from build123d import *

# Parameters (mm, degrees)
CROQUIS1_W              = 220
CROQUIS1_H              = 320
CROQUIS1_R              = 1.55
CROQUIS1_R_2            = 1.575
SALIENTE_EXTRUIR1_DEPTH = 3
CROQUIS2_OUTSIDE_W      = 299.668
CROQUIS2_OUTSIDE_H      = 399.668
CORTAR_EXTRUIR1_DEPTH   = 3
REDONDEO1_R             = 3


with BuildPart() as part:
    # Croquis1 → Saliente-Extruir1 (new body)
    with BuildSketch(Plane(origin=(0, 0, 0), x_dir=(1, 0, 0), z_dir=(0, 1, 0))):
        with Locations((110, 160)):
            Rectangle(CROQUIS1_W, CROQUIS1_H)
        with Locations((185, 167.5)):
            Circle(CROQUIS1_R, mode=Mode.SUBTRACT)
        with Locations((205, 167.5)):
            Circle(CROQUIS1_R, mode=Mode.SUBTRACT)
        with Locations((185, 152.5)):
            Circle(CROQUIS1_R, mode=Mode.SUBTRACT)
        with Locations((205, 152.5)):
            Circle(CROQUIS1_R, mode=Mode.SUBTRACT)
        with Locations((35, 215.5)):
            Circle(CROQUIS1_R_2, mode=Mode.SUBTRACT)
        with Locations((35, 200.5)):
            Circle(CROQUIS1_R_2, mode=Mode.SUBTRACT)
        with Locations((35, 119.5)):
            Circle(CROQUIS1_R_2, mode=Mode.SUBTRACT)
        with Locations((35, 104.5)):
            Circle(CROQUIS1_R_2, mode=Mode.SUBTRACT)
        with Locations((5.5, 314.5)):
            Circle(CROQUIS1_R_2, mode=Mode.SUBTRACT)
        with Locations((214.5, 314.5)):
            Circle(CROQUIS1_R_2, mode=Mode.SUBTRACT)
        with Locations((214.5, 5.5)):
            Circle(CROQUIS1_R_2, mode=Mode.SUBTRACT)
        with Locations((5.5, 5.5)):
            Circle(CROQUIS1_R_2, mode=Mode.SUBTRACT)
        with Locations((15, 200.5)):
            Circle(CROQUIS1_R_2, mode=Mode.SUBTRACT)
        with Locations((15, 215.5)):
            Circle(CROQUIS1_R_2, mode=Mode.SUBTRACT)
        with Locations((15, 104.5)):
            Circle(CROQUIS1_R_2, mode=Mode.SUBTRACT)
        with Locations((15, 119.5)):
            Circle(CROQUIS1_R_2, mode=Mode.SUBTRACT)
        with Locations((110, 180)):
            Circle(CROQUIS1_R_2, mode=Mode.SUBTRACT)
        with Locations((110, 140)):
            Circle(CROQUIS1_R_2, mode=Mode.SUBTRACT)
        with Locations((185, 104.5)):
            Circle(CROQUIS1_R_2, mode=Mode.SUBTRACT)
        with Locations((205, 104.5)):
            Circle(CROQUIS1_R_2, mode=Mode.SUBTRACT)
        with Locations((205, 119.5)):
            Circle(CROQUIS1_R_2, mode=Mode.SUBTRACT)
        with Locations((185, 119.5)):
            Circle(CROQUIS1_R_2, mode=Mode.SUBTRACT)
        with Locations((185, 200.5)):
            Circle(CROQUIS1_R_2, mode=Mode.SUBTRACT)
        with Locations((185, 215.5)):
            Circle(CROQUIS1_R_2, mode=Mode.SUBTRACT)
        with Locations((205, 200.5)):
            Circle(CROQUIS1_R_2, mode=Mode.SUBTRACT)
        with Locations((205, 215.5)):
            Circle(CROQUIS1_R_2, mode=Mode.SUBTRACT)
        with Locations((5.5, 160)):
            Circle(CROQUIS1_R_2, mode=Mode.SUBTRACT)
        with Locations((35, 152.5)):
            Circle(CROQUIS1_R, mode=Mode.SUBTRACT)
        with Locations((15, 152.5)):
            Circle(CROQUIS1_R, mode=Mode.SUBTRACT)
        with Locations((15, 167.5)):
            Circle(CROQUIS1_R, mode=Mode.SUBTRACT)
        with Locations((35, 167.5)):
            Circle(CROQUIS1_R, mode=Mode.SUBTRACT)
        with Locations((214.5, 160)):
            Circle(CROQUIS1_R_2, mode=Mode.SUBTRACT)
    extrude(amount=SALIENTE_EXTRUIR1_DEPTH)

    # Croquis2 outside → Cortar-Extruir1 (cut)
    with BuildSketch(Plane(origin=(0, 3, 0), x_dir=(1, 0, 0), z_dir=(0, 1, 0))):
        with Locations((110, 160)):
            Rectangle(CROQUIS2_OUTSIDE_W, CROQUIS2_OUTSIDE_H)
        with BuildLine():
            Line((9, 148.77502784), (9, 94.5))
            Line((9, 94.5), (19, 94.5))
            Line((19, 94.5), (19, 30))
            Line((19, 30), (1.298802547, 9.049639413))
            ThreePointArc((1.298802547, 9.049639413), (1.950360587, 1.298802547), (9.701197453, 1.950360587))
            Line((9.701197453, 1.950360587), (24.106631311, 19))
            Line((24.106631311, 19), (195.893368689, 19))
            Line((195.893368689, 19), (210.298802547, 1.950360587))
            ThreePointArc((210.298802547, 1.950360587), (218.049639413, 1.298802547), (218.701197453, 9.049639413))
            Line((218.701197453, 9.049639413), (201, 30))
            Line((201, 30), (201, 94.5))
            Line((201, 94.5), (211, 94.5))
            Line((211, 94.5), (211, 148.77502784))
            ThreePointArc((211, 148.77502784), (212.318863014, 152.528287293), (215.695652174, 154.631535054))
            ThreePointArc((215.695652174, 154.631535054), (220, 160), (215.695652174, 165.368464946))
            ThreePointArc((215.695652174, 165.368464946), (212.318863014, 167.471712707), (211, 171.22497216))
            Line((211, 171.22497216), (211, 225.5))
            Line((211, 225.5), (201, 225.5))
            Line((201, 225.5), (201, 290))
            Line((201, 290), (218.701197453, 310.950360587))
            ThreePointArc((218.701197453, 310.950360587), (218.049639413, 318.701197453), (210.298802547, 318.049639413))
            Line((210.298802547, 318.049639413), (195.893368689, 301))
            Line((195.893368689, 301), (24.106631311, 301))
            Line((24.106631311, 301), (9.701197453, 318.049639413))
            ThreePointArc((9.701197453, 318.049639413), (1.950360587, 318.701197453), (1.298802547, 310.950360587))
            Line((1.298802547, 310.950360587), (19, 290))
            Line((19, 290), (19, 225.5))
            Line((19, 225.5), (9, 225.5))
            Line((9, 225.5), (9, 171.22497216))
            ThreePointArc((9, 171.22497216), (7.681136986, 167.471712707), (4.304347826, 165.368464946))
            ThreePointArc((4.304347826, 165.368464946), (0, 160), (4.304347826, 154.631535054))
            ThreePointArc((4.304347826, 154.631535054), (7.681136986, 152.528287293), (9, 148.77502784))
        make_face(mode=Mode.SUBTRACT)
        with BuildLine():
            Line((182, 276), (182, 246))
            ThreePointArc((182, 246), (179.071067812, 238.928932188), (172, 236))
            Line((172, 236), (118, 236))
            ThreePointArc((118, 236), (116.585786438, 236.585786438), (116, 238))
            Line((116, 238), (116, 284))
            ThreePointArc((116, 284), (116.585786438, 285.414213562), (118, 286))
            Line((118, 286), (172, 286))
            ThreePointArc((172, 286), (179.071067812, 283.071067812), (182, 276))
        make_face()
        with BuildLine():
            Line((102, 286), (48, 286))
            ThreePointArc((48, 286), (40.928932188, 283.071067812), (38, 276))
            Line((38, 276), (38, 246))
            ThreePointArc((38, 246), (40.928932188, 238.928932188), (48, 236))
            Line((48, 236), (102, 236))
            ThreePointArc((102, 236), (103.414213562, 236.585786438), (104, 238))
            Line((104, 238), (104, 284))
            ThreePointArc((104, 284), (103.414213562, 285.414213562), (102, 286))
        make_face()
        with BuildLine():
            Line((102, 84), (48, 84))
            ThreePointArc((48, 84), (40.928932188, 81.071067812), (38, 74))
            Line((38, 74), (38, 44))
            ThreePointArc((38, 44), (40.928932188, 36.928932188), (48, 34))
            Line((48, 34), (102, 34))
            ThreePointArc((102, 34), (103.414213562, 34.585786438), (104, 36))
            Line((104, 36), (104, 82))
            ThreePointArc((104, 82), (103.414213562, 83.414213562), (102, 84))
        make_face()
        with BuildLine():
            Line((116, 36), (116, 82))
            ThreePointArc((116, 82), (116.585786438, 83.414213562), (118, 84))
            Line((118, 84), (172, 84))
            ThreePointArc((172, 84), (179.071067812, 81.071067812), (182, 74))
            Line((182, 74), (182, 44))
            ThreePointArc((182, 44), (179.071067812, 36.928932188), (172, 34))
            Line((172, 34), (118, 34))
            ThreePointArc((118, 34), (116.585786438, 34.585786438), (116, 36))
        make_face()
        with BuildLine():
            Line((55, 152), (55, 119))
            ThreePointArc((55, 119), (57.928932188, 111.928932188), (65, 109))
            Line((65, 109), (85, 109))
            ThreePointArc((85, 109), (92.071067812, 111.928932188), (95, 119))
            Line((95, 119), (95, 152))
            ThreePointArc((95, 152), (94.414213562, 153.414213562), (93, 154))
            Line((93, 154), (57, 154))
            ThreePointArc((57, 154), (55.585786438, 153.414213562), (55, 152))
        make_face()
        with BuildLine():
            Line((93, 166), (57, 166))
            ThreePointArc((57, 166), (55.585786438, 166.585786438), (55, 168))
            Line((55, 168), (55, 201))
            ThreePointArc((55, 201), (57.928932188, 208.071067812), (65, 211))
            Line((65, 211), (85, 211))
            ThreePointArc((85, 211), (92.071067812, 208.071067812), (95, 201))
            Line((95, 201), (95, 168))
            ThreePointArc((95, 168), (94.414213562, 166.585786438), (93, 166))
        make_face()
        with BuildLine():
            Line((135, 109), (155, 109))
            ThreePointArc((155, 109), (162.071067812, 111.928932188), (165, 119))
            Line((165, 119), (165, 152))
            ThreePointArc((165, 152), (164.414213562, 153.414213562), (163, 154))
            Line((163, 154), (127, 154))
            ThreePointArc((127, 154), (125.585786438, 153.414213562), (125, 152))
            Line((125, 152), (125, 119))
            ThreePointArc((125, 119), (127.928932188, 111.928932188), (135, 109))
        make_face()
        with BuildLine():
            Line((127, 166), (163, 166))
            ThreePointArc((163, 166), (164.414213562, 166.585786438), (165, 168))
            Line((165, 168), (165, 201))
            ThreePointArc((165, 201), (162.071067812, 208.071067812), (155, 211))
            Line((155, 211), (135, 211))
            ThreePointArc((135, 211), (127.928932188, 208.071067812), (125, 201))
            Line((125, 201), (125, 168))
            ThreePointArc((125, 168), (125.585786438, 166.585786438), (127, 166))
        make_face()
    extrude(amount=-CORTAR_EXTRUIR1_DEPTH, mode=Mode.SUBTRACT)

    # Redondeo1
    redondeo1_edges = [part.edges().sort_by_distance(p)[0] for p in [
        (19, 1.5, -94.5),
        (9, 1.5, -94.5),
        (9, 1.5, -225.5),
        (19, 1.5, -225.5),
        (19, 1.5, -290),
        (24.106631311, 1.5, -301),
        (195.893368689, 1.5, -301),
        (201, 1.5, -290),
        (201, 1.5, -225.5),
        (211, 1.5, -225.5),
        (211, 1.5, -94.5),
        (201, 1.5, -94.5),
        (201, 1.5, -30),
        (195.893368689, 1.5, -19),
        (24.106631311, 1.5, -19),
        (19, 1.5, -30),
    ]]
    fillet(redondeo1_edges, radius=REDONDEO1_R)


solid = part.part
Geometry: final body of the model. Coordinates: model frame, mm. A direction names the side the tool comes from. Give positions to 0.01 mm unless a question says otherwise; leave off trailing zeros. Loops run counter-clockwise (first coordinate to the right, second up) from the corner with the lowest first, then second, coordinate; pieces in that order, holes last. Notation, with made-up numbers: (57.5, -25) -> (93.5, -25) arc R32 cw to (93.5, 13) -> close; hole circle Ø3 at (52.25, 58.25). An arc over 180 degrees is marked (long way). Put each result on its own line as item: value.
1. Cut plane B-B (y = 0.5). Count the separate pieces of the cut face and the enclosed holes in it, plus the area to 3 significant figures.
Taken from the geometry:
separate pieces: 1
enclosed holes: 40
area: 35,000 mm2
2. Set-up query: faces 4 (the flat face through (16.549, 1.521, -309.945)), 5 (the flat face through (9.914, 1.521, -19.246)), 6 (the cylindrical face through (91.99, 1.52, -208.15)). Return all of +Z, -Z, +X, -X, +Y, -Y with unobstructed straight access to the full face (end or side cutting, diameter ignored); none if empty.
Taken from the geometry:
face 4: -Z, +Y, -Y
face 5: -X, +Y, -Y
face 6: +Y, -Y
3. Pull-direction query (Z, two-part tool) for faces 1 (the cylindrical face through (179.15, 1.52, -37.01)), 2 (the flat face through (203.64, 1.52, -310.17)), 3 (the flat face through (108, 3, -127)); classes: released by +Z, released by -Z, zero draft, split by the parting line, or undercut.
Taken from the geometry:
face 1: undercut
face 2: released by -Z
face 3: zero draft
4. Cut plane A-A (z = -77.5). Return the cut outline in (x, y).
Taken from the geometry:
outline: (19, 0) -> (38.63, 0) -> (38.63, 3) -> (19, 3) -> close; (104, 0) -> (116, 0) -> (116, 3) -> (104, 3) -> close; (181.37, 0) -> (201, 0) -> (201, 3) -> (181.37, 3) -> close
5. Pin query (flat end, axial travel): P1, Ø1.5, axis at x = 96, y = 1.5, coming from the +Z side; P2, Ø10, axis at x = 183, z = -186, coming from the -Y side; P3, Ø1.5, axis at x = 26, y = 2.5, coming from the -Z side; P4, Ø1.5, axis at y = 1, z = -135.5, coming from the -X side. Return the tip coordinate at first contact, or that it passes through.
Taken from the geometry:
P1: stops at z = -19
P2: stops at y = 0
P3: stops at z = -301.01
P4: stops at x = 9
6. Ray query, line 1 along Z through (x, y) = (64, 2.8); line 2 along Z through (x, y) = (166.5, 2.1); line 3 along Z through (x, y) = (110, 0.7) (3 decimals). Return the intervals inside material, ascending. Write a range as [from, to].
Taken from the geometry:
line 1: z = [-301, -286], [-236, -210.95], [-166, -154], [-109.05, -84], [-34, -19]
line 2: z = [-301, -286], [-236, -84], [-34, -19]
line 3: z = [-301, -181.575], [-178.425, -141.575], [-138.425, -19]
